Can you work these out from the model? Positions are in its coordinate system, mm. A direction names the side the tool comes from. Give positions to 0.01 mm unless a question says otherwise; leave off trailing zeros. Write each loop counter-clockwise with the first axis right and the second up, starting at its lowest first coordinate (ties: lowest second). Pieces come first, ordered by that corner, then holes.
```python
from build123d import *

# Parameters (mm, degrees)
SKETCH1_W               = 19
SKETCH1_H               = 19
SKETCH1_W_2             = 17
SKETCH1_H_2             = 17
BOSS_EXTRUDE1_DEPTH     = 280
CUT_EXTRUDE3_DEPTH      = 1
CUT_EXTRUDE3_DEPTH_BACK = 20
CUT_EXTRUDE4_DEPTH      = 1
CUT_EXTRUDE4_DEPTH_BACK = 20


with BuildPart() as part:
    # Sketch1 → Boss-Extrude1 (new body)
    with BuildSketch(Plane.XY):
        Rectangle(SKETCH1_W, SKETCH1_H)
        Rectangle(SKETCH1_W_2, SKETCH1_H_2, mode=Mode.SUBTRACT)
    extrude(amount=BOSS_EXTRUDE1_DEPTH)

    # Sketch4 → Cut-Extrude3 (cut, two sides)
    with BuildSketch(Plane(origin=(9.5, 0, 0), x_dir=(0, 0, -1), z_dir=(1, 0, 0))) as cut_extrude3_sk:
        Polygon((-565.643902481, -504.24975197), (-280, -9.5), (-269.030344885, 9.5), (16.613557596, 504.24975197), (-972.885946344, 1075.537556933), (-1555.143406422, 67.038052993), align=None)
    extrude(amount=CUT_EXTRUDE3_DEPTH, mode=Mode.SUBTRACT)
    extrude(cut_extrude3_sk.sketch, amount=-CUT_EXTRUDE3_DEPTH_BACK, mode=Mode.SUBTRACT)

    # Sketch5 → Cut-Extrude4 (cut, two sides)
    with BuildSketch(Plane(origin=(9.5, 0, 0), x_dir=(0, 0, -1), z_dir=(1, 0, 0))) as cut_extrude4_sk:
        Polygon((285.643902481, -504.24975197), (0, -9.5), (-10.969655115, 9.5), (-296.613557596, 504.24975197), (692.885946344, 1075.537556933), (1275.143406422, 67.038052993), align=None)
    extrude(amount=CUT_EXTRUDE4_DEPTH, mode=Mode.SUBTRACT)
    extrude(cut_extrude4_sk.sketch, amount=-CUT_EXTRUDE4_DEPTH_BACK, mode=Mode.SUBTRACT)


solid = part.part
```
1) If we mould it in two halves opening along Y, with no side actions, what happens to faces 3 (the face through (-9.5, 0, 138)), 4 (the face through (0, 9.5, 138)), 5 (the face through (-8.5, 0, 138)), 6 (the face through (0, -9.5, 138))? For each: +Y half, -Y half, draft (parallel to the pull), parting line (faces both ways), or undercut.
Values follow:
face 3: draft
face 4: +Y half
face 5: undercut
face 6: -Y half
2) For pin 1 Ø4 at (x, y) = (-2, -7) entering from +Z, with a flat end and sliding along its axis, tell me the tip position at first contact or that it passes through.
Values follow:
pin 1: stops at z = 279.71
3) Suppose I cut it at C-C on z = 172. Write out the boundary of the cut face in (x, y).
Values follow:
outline: (-9.5, -9.5) - (9.5, -9.5) - (9.5, 9.5) - (-9.5, 9.5) - close; hole (-8.5, -8.5) - (8.5, -8.5) - (8.5, 8.5) - (-8.5, 8.5) - close
4) Please list where these lines run through material, in increasing order: L1, parallel to X at y = 3.75, z = 268; L2, parallel to Z at x = -2, y = 8.75.
Values follow:
L1: x = -9.5 to -8.5, 8.5 to 9.5
L2: z = 10.54 to 269.46
5) Suppose I cut it at A-A on x = -2.5. Write out the boundary of the cut face in (y, z), plus the area to 3 significant figures.
Values follow:
outline: (-9.5, 0) - (-8.5, 0.58) - (-8.5, 279.42) - (-9.5, 280) - close; (8.5, 10.39) - (9.5, 10.97) - (9.5, 269.03) - (8.5, 269.61) - close
area: 538 mm2
6) For faces 1 (the face through (0, -8.5, 138)), 2 (the face through (-9.1, -0.75, 274.95)), which set-ups out of +Z, -Z, +X, -X, +Y, -Y let a thin tool reach every point of the face, with its end or its side?
Values follow:
face 1: +Z, -Z
face 2: +Z, +X, -X, +Y
7) Suppose I cut it at B-B on y = 0.75. Write out the boundary of the cut face in (x, z).
Values follow:
outline: (-9.5, 5.92) - (-8.5, 5.92) - (-8.5, 274.08) - (-9.5, 274.08) - close; (8.5, 5.92) - (9.5, 5.92) - (9.5, 274.08) - (8.5, 274.08) - close
